For this review, use the dimensioned drawing (mm, ordinates from the lowest corner) and the shaded views. A direction names the side the tool comes from. Coordinates: 2 decimals unless noted, no trailing zeros. Loops run counter-clockwise (first coordinate to the right, second up) from the corner with the lowest first, then second, coordinate; pieces in that order, holes last. Notation, with made-up numbers: M -3,-21 L 38,-21 A26 ccw 38,0 Z; hole C 57,-7 d3. An arc over 180 degrees is marked long. One line per item, written item: value.
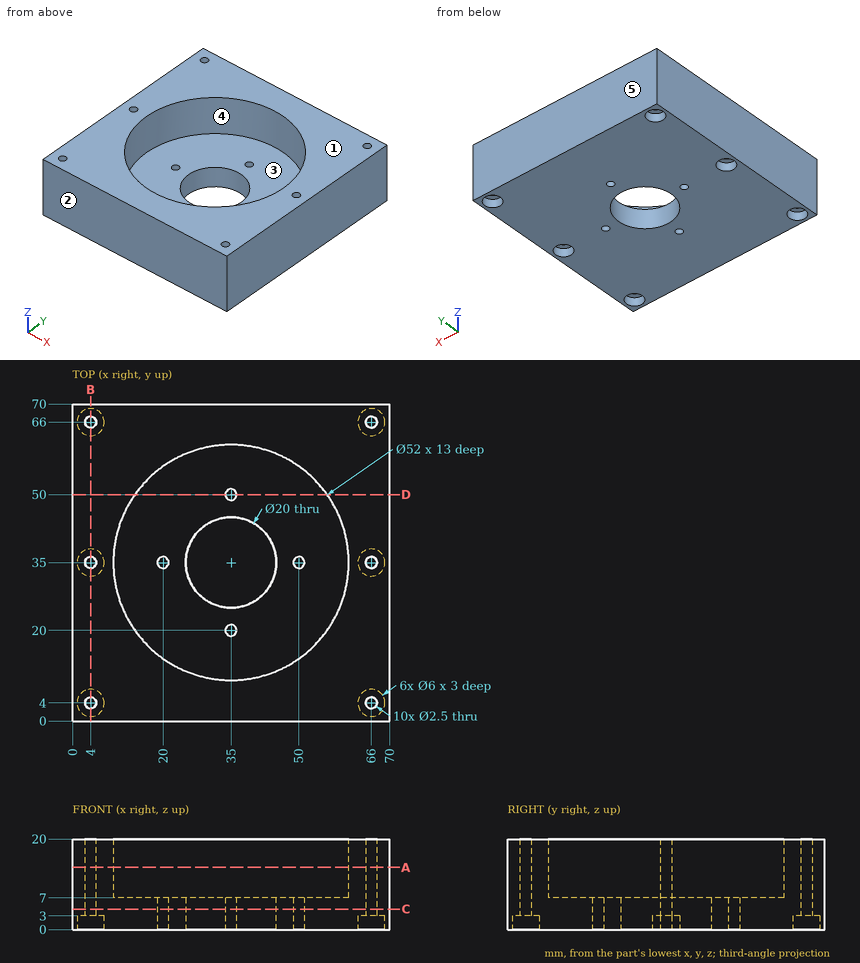
(1) Tool access review of the marked faces 4 and 5: name each direction out of +Z, -Z, +X, -X, +Y, -Y from which nothing blocks a thin tool from reaching the whole face with its end or side.
Checks:
face 4: +Z
face 5: +Z, -Z, +X, -X, +Y
(2) Add section B-B on x = 4. State the section outline as (y, z) points.
Checks:
outline: M 0,0 L 1,0 L 1,3 L 2.75,3 L 2.75,20 L 0,20 Z; M 5.25,3 L 7,3 L 7,0 L 32,0 L 32,3 L 33.75,3 L 33.75,20 L 5.25,20 Z; M 36.25,3 L 38,3 L 38,0 L 63,0 L 63,3 L 64.75,3 L 64.75,20 L 36.25,20 Z; M 67.25,3 L 69,3 L 69,0 L 70,0 L 70,20 L 67.25,20 Z
(3) Add section A-A on z = 13.75. State the section outline as (x, y) points.
Checks:
outline: M 0,0 L 70,0 L 70,70 L 0,70 Z; hole C 4,4 d2.5; hole C 4,35 d2.5; hole C 4,66 d2.5; hole C 35,35 d52; hole C 66,4 d2.5; hole C 66,35 d2.5; hole C 66,66 d2.5
(4) Insertion check: pin 1 Ø15.5 at (x, y) = (45, 42.5) entering from +Z. The pin has a flat end and moves straight along its axis. Give the tip position at first contact, or say it passes through.
Checks:
pin 1: z = 7
(5) Add section D-D on y = 50. State the section outline as (x, z) points, then the cut area to 3 significant figures.
Checks:
outline: M 0,0 L 33.75,0 L 33.75,7 L 13.76,7 L 13.76,20 L 0,20 Z; M 36.25,0 L 70,0 L 70,20 L 56.24,20 L 56.24,7 L 36.25,7 Z
area: 830 mm^2
(6) Draft analysis for pull direction Y (two halves, no side actions). For the marked faces 1, 2 and 3, state which applies: pulls with the +Y half, pulls with the -Y half, needs draft (parallel to the pull), parting line crosses it, or undercut.
Checks:
face 1: needs draft
face 2: pulls with the -Y half
face 3: undercut
(7) To check wall thickness, follow L1, parallel to X at y = 4, z = 10.25; L2, parallel to Y at x = 4, z = 14.25; L3, parallel to Y at x = 4, z = 1.6. State the ranges of each line that lie inside material, in increasing order. Write a range as [from, to].
Checks:
L1: [0, 2.75], [5.25, 64.75], [67.25, 70]
L2: [0, 2.75], [5.25, 33.75], [36.25, 64.75], [67.25, 70]
L3: [0, 1], [7, 32], [38, 63], [69, 70]
(8) Add section C-C on z = 4.5. State how many separate pieces and enclosed holes the cut face has, then the cut area to 3 significant figures.
Checks:
separate pieces: 1
enclosed holes: 11
area: 4,540 mm^2
